from build123d import *

# Parameters (mm, degrees)
SKETCH17_R                                        = 43.5
BOSS_EXTRUDE1_DEPTH                               = 5
SKETCH19_R                                        = 43.5
SKETCH19_R_2                                      = 38.5
BOSS_EXTRUDE2_DEPTH                               = 35
SKETCH20_R                                        = 20.5
CUT_EXTRUDE1_DEPTH                                = 5
SKETCH26_W                                        = 170
SKETCH26_H                                        = 60
BOSS_EXTRUDE3_DEPTH                               = 5
BOSS_EXTRUDE4_DEPTH                               = 40
CSK_FOR_3_FLAT_HEAD_MACHINE_SCREW_100_D           = 2.794
CSK_FOR_3_FLAT_HEAD_MACHINE_SCREW_100_CSINK_D     = 5.0546
CSK_FOR_3_FLAT_HEAD_MACHINE_SCREW_100_CSINK_ANGLE = 100
CUT_EXTRUDE2_DEPTH                                = 40


with BuildPart() as part:
    # Sketch17 → Boss-Extrude1 (new body)
    with BuildSketch(Plane.XY):
        Circle(SKETCH17_R)
    extrude(amount=BOSS_EXTRUDE1_DEPTH)

    # Sketch19 → Boss-Extrude2 (add)
    with BuildSketch(Plane.XY.offset(5)):
        Circle(SKETCH19_R)
        Circle(SKETCH19_R_2, mode=Mode.SUBTRACT)
    extrude(amount=BOSS_EXTRUDE2_DEPTH)

    # Sketch20 → Cut-Extrude1 (cut)
    with BuildSketch(Plane(origin=(0, 0, 0), x_dir=(-1, 0, 0), z_dir=(0, 0, -1))):
        Circle(SKETCH20_R)
    extrude(amount=-CUT_EXTRUDE1_DEPTH, mode=Mode.SUBTRACT)

    # Sketch26 → Boss-Extrude3 (add)
    with BuildSketch(Plane(origin=(0, -43.5, 0), x_dir=(1, 0, 0), z_dir=(0, 1, 0))):
        with Locations((0, -20)):
            Rectangle(SKETCH26_W, SKETCH26_H)
    extrude(amount=BOSS_EXTRUDE3_DEPTH)

    # Sketch27 → Boss-Extrude4 (add)
    with BuildSketch(Plane.XY.offset(40)):
        Polygon((-85, -38.5), (-32.53104334, 28.878732991), (-42.379072789, 9.811431574), (-80, -38.5), align=None)
        Polygon((32.53104334, 28.878732991), (42.379072789, 9.811431574), (80, -38.5), (85, -38.5), align=None)
    extrude(amount=-BOSS_EXTRUDE4_DEPTH)

    # CSK for #3 Flat Head Machine Screw (100)4 (through all)
    with Locations(Plane(origin=(0, 0, 0), x_dir=(-1, 0, 0), z_dir=(0, 0, -1))):
        with Locations((-24.248711306, 14), (-15, 25.980762114), (24.248711306, 14), (30, 0), (0, -28), (-15, -25.980762114)):
            CounterSinkHole(CSK_FOR_3_FLAT_HEAD_MACHINE_SCREW_100_D / 2, CSK_FOR_3_FLAT_HEAD_MACHINE_SCREW_100_CSINK_D / 2, counter_sink_angle=CSK_FOR_3_FLAT_HEAD_MACHINE_SCREW_100_CSINK_ANGLE)

    # Sketch34 → Cut-Extrude2 (cut)
    with BuildSketch(Plane(origin=(0, 43.5, 0), x_dir=(1, 0, 0), z_dir=(0, 1, 0))):
        with BuildLine():
            Line((-25, -40), (25, -40))
            Line((25, -40), (25, -30))
            ThreePointArc((25, -30), (23.535533906, -26.464466094), (20, -25))
            Line((20, -25), (-20, -25))
            ThreePointArc((-20, -25), (-23.535533906, -26.464466094), (-25, -30))
            Line((-25, -30), (-25, -40))
        make_face()
    extrude(amount=-CUT_EXTRUDE2_DEPTH, mode=Mode.SUBTRACT)


solid = part.part
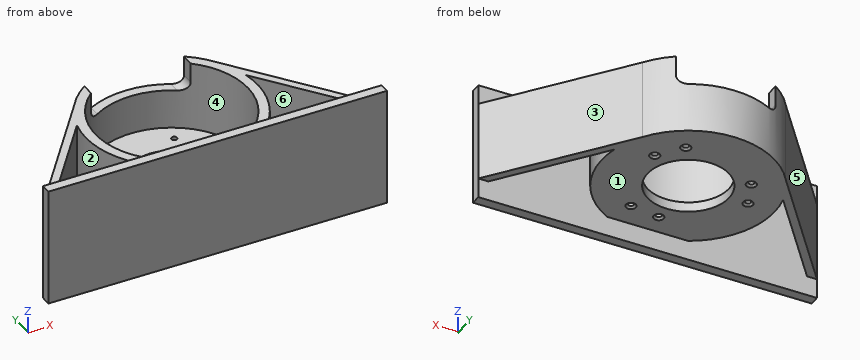
Work out the finished part from the listing and answer in its coordinate system (mm). Face numbers are marked on the shaded views. A direction names the side the tool comes from. Give positions to 0.01 mm unless a question says otherwise; leave off trailing zeros. Loops run counter-clockwise (first coordinate to the right, second up) from the corner with the lowest first, then second, coordinate; pieces in that order, holes last. Notation, with made-up numbers: (46, 3.25) - (63, 3.25) arc R20 ccw to (63, 26.25) - close; hole circle Ø9 at (5.5, 36.25). An arc over 180 degrees is marked (long way). Answer in a Markdown table with one row per item. Add a question column.
Q1. The part is cut by section A-A (z = 17). Determine the outline of the cut face in (x, y), and give its area (3 significant figures).
Q2. Determine the mould class of the marked faces 1, 2 and 3 for opening direction Y: released by +Y, released by -Y, zero draft, split by the parting line, or undercut.
Q3. The part is cut by section C-C (z = 46). Determine the outline of the cut face in (x, y).
Q4. Each of these flat-tipped pins is pushed along its axis until it touches: P1, Ø2.5, axis at x = 0, y = -28, coming from the -Z side; P2, Ø1.5, axis at x = 9.5, z = 9, coming from the +Y side; P3, Ø5, axis at y = 32.5, z = 35, coming from the -X side; P4, Ø10, axis at y = 11.5, z = 31.5, coming from the -X side. Where does it stop, or does it pass through?
Q5. A tool of negligible diameter and unlimited length cuts with its end or side. For the marked faces 4, 5 and 6, from which of +Z, -Z, +X, -X, +Y, -Y can it reach the whole face along a straight path? Write none if from no direction.
Q6. The part is cut by section B-B (x = 73.5). Determine the outline of the cut face in (y, z).
Q7. Consider line 1 along Y through (x, z) = (0, 1.15); line 2 along Y through (x, z) = (-33, 17.5); line 3 along Y through (x, z) = (15, 3.85). Determine where each line is inside the solid, lowest interval first.
Solution:
| question | item | result |
|---|---|---|
| 1 | outline | (-85, -43.5) - (85, -43.5) - (85, -38.5) - (35.97, 24.46) arc R43.5 ccw to (-35.97, 24.46) - (-85, -38.5) - close; hole (-80, -38.5) - (-20.25, -38.5) arc R43.5 cw to (-42.38, 9.81) - close; hole circle Ø77 at (0, 0); hole (20.25, -38.5) - (80, -38.5) - (42.38, 9.81) arc R43.5 cw to start |
| 1 | area | 2,540 mm² |
| 2 | face 1 | zero draft |
| 2 | face 2 | undercut |
| 2 | face 3 | released by +Y |
| 3 | outline | (-85, -43.5) - (85, -43.5) - (85, -38.5) - (-85, -38.5) - close |
| 4 | P1 | passes through |
| 4 | P2 | stops at y = 42.61 |
| 4 | P3 | stops at x = -31.5 |
| 4 | P4 | stops at x = -49.96 |
| 5 | face 4 | +Z |
| 5 | face 5 | +Z, -Z, -X, +Y |
| 5 | face 6 | +Z, -Z |
| 6 | outline | (-43.5, -10) - (-38.5, -10) - (-38.5, 50) - (-43.5, 50) - close; (-30.15, 0) - (-23.73, 0) - (-23.73, 40) - (-30.15, 40) - close |
| 7 | line 1 | y = -43.5 to -29.4, -26.6 to -20.5, 20.5 to 43.5 |
| 7 | line 2 | y = -43.5 to -38.5, -28.34 to -19.83, 19.83 to 28.34 |
| 7 | line 3 | y = -43.5 to -27.38, -24.58 to -13.97, 13.97 to 24.58, 27.38 to 40.83 |
